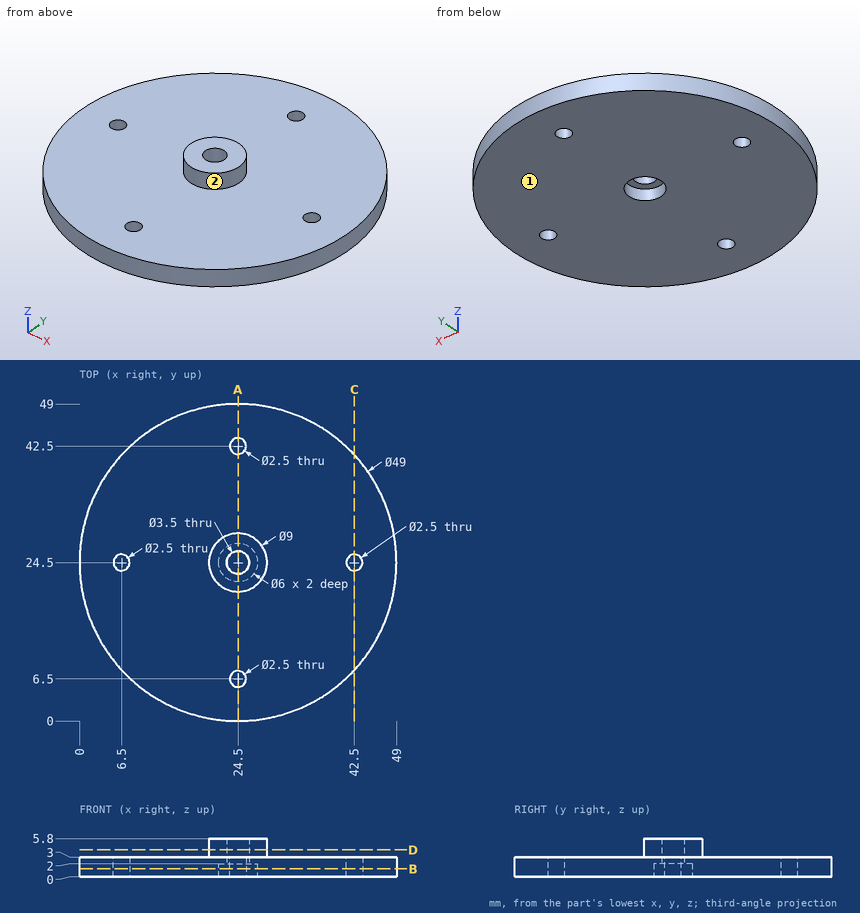
Could you check a few things on this drawing? It's one solid part, dimensions in mm from its lowest x, y, z. A direction names the side the tool comes from. Coordinates: 2 decimals unless noted, no trailing zeros. Order: outer loops, then holes, each group sorted by start corner. A loop starts at its lowest first (then second) coordinate and runs counter-clockwise, first axis right, second up. Notation, with made-up numbers: M 24.25,-6 L 33.25,-6 A13 cw 33.25,17 Z; hole C 58,-11.75 d4. An arc over 180 degrees is marked long. Answer as a JSON object with one key per item and string values. Group by question number.
(1) Which directions (+Z, -Z, +X, -X, +Y, -Y) give clear straight access to the entire face, cutting with the end or side of a thin tool? Please do the marked faces 1 and 2.
(2) Suppose I cut it at B-B, the plane z = 1.2. Please give me the cut outline in (x, y), then the cut area to 3 significant figures.
(3) Suppose I cut it at A-A, the plane x = 24.5. Please give me the cut outline in (y, z).
(4) For pin 1 (5 mm diameter, centred on x = 24.5, y = 24.5, fed in from +Z); pin 2 (1.8 mm diameter, centred on x = 26, y = 24, fed in from -Z); pin 3 (14.5 mm diameter, centred on x = 15, y = 33.5, fed in from +Z); pin 4 (1 mm diameter, centred on y = 26.5, z = 2, fed in from -X), each with a flat end and sliding along its axis, tell me the tip position at first contact or that it passes through.
(5) Suppose I cut it at D-D, the plane z = 4.1. Please give me the cut outline in (x, y).
(6) Suppose I cut it at C-C, the plane x = 42.5. Please give me the cut outline in (y, z).
(7) I need wall thicknesses on probe 1 along Y at (x, z) = (24.5, 5.05); probe 2 along Y at (x, z) = (24.5, 1.3); probe 3 along Y at (x, z) = (25, 2.1). Which ranges of each line are inside material? Lowest first, please.
Values found:
{
 "1": {"face 1": "-Z, +X, -X, +Y, -Y", "face 2": "+Z"},
 "2": {"outline": "C 24.5,24.5 d49; hole C 6.5,24.5 d2.5; hole C 24.5,24.5 d6; hole C 24.5,6.5 d2.5; hole C 24.5,42.5 d2.5; hole C 42.5,24.5 d2.5", "area": "1,840 mm^2"},
 "3": {"outline": "M 0,0 L 5.25,0 L 5.25,3 L 0,3 Z; M 7.75,0 L 21.5,0 L 21.5,2 L 22.75,2 L 22.75,5.8 L 20,5.8 L 20,3 L 7.75,3 Z; M 26.25,2 L 27.5,2 L 27.5,0 L 41.25,0 L 41.25,3 L 29,3 L 29,5.8 L 26.25,5.8 Z; M 43.75,0 L 49,0 L 49,3 L 43.75,3 Z"},
 "4": {"pin 1": "stops at z = 5.8", "pin 2": "stops at z = 2", "pin 3": "stops at z = 3", "pin 4": "stops at x = 0.05"},
 "5": {"outline": "C 24.5,24.5 d9; hole C 24.5,24.5 d3.5"},
 "6": {"outline": "M 7.88,0 L 23.25,0 L 23.25,3 L 7.88,3 Z; M 25.75,0 L 41.12,0 L 41.12,3 L 25.75,3 Z"},
 "7": {"probe 1": "y = 20 to 22.75, 26.25 to 29", "probe 2": "y = 0 to 5.25, 7.75 to 21.5, 27.5 to 41.25, 43.75 to 49", "probe 3": "y = 0.01 to 5.35, 7.65 to 22.82, 26.18 to 41.35, 43.65 to 48.99"}
}
